```python
from build123d import *

# Parameters (mm, degrees)
BOSS_EXTRUDE1_DEPTH = 5.9944
SKETCH2_R           = 4.7244
CUT_EXTRUDE1_DEPTH  = 6.9944
SKETCH3_W           = 38.1
SKETCH3_H           = 1.5875
CUT_EXTRUDE2_DEPTH  = 6.9944


with BuildPart() as part:
    # Sketch1 → Boss-Extrude1 (new body)
    with BuildSketch(Plane.XY):
        Polygon((0, 0), (-38.1, 0), (-38.1, 6.35), (-44.0944, 6.35), (-44.0944, 19.05), (-38.1, 19.05), (-38.1, 31.75), (-44.0944, 31.75), (-44.0944, 44.45), (-38.1, 44.45), (-38.1, 50.8), (0, 50.8), (0, 44.45), (5.9944, 44.45), (5.9944, 31.75), (0, 31.75), (0, 19.05), (5.9944, 19.05), (5.9944, 6.35), (0, 6.35), align=None)
    extrude(amount=BOSS_EXTRUDE1_DEPTH)

    # Sketch2 → Cut-Extrude1 (cut, through all)
    with BuildSketch(Plane.XY.offset(5.9944)):
        with Locations((-19.05, 31.75)):
            Circle(SKETCH2_R)
    extrude(amount=-CUT_EXTRUDE1_DEPTH, mode=Mode.SUBTRACT)

    # Sketch3 → Cut-Extrude2 (cut, through all)
    with BuildSketch(Plane.XY.offset(5.9944)):
        with Locations((-19.05, 0.79375)):
            Rectangle(SKETCH3_W, SKETCH3_H)
        with Locations((-19.05, 50.00625)):
            Rectangle(SKETCH3_W, SKETCH3_H)
    extrude(amount=-CUT_EXTRUDE2_DEPTH, mode=Mode.SUBTRACT)


solid = part.part
```
Source: CAD feature listing. Evaluate the final solid. Frame: model axes, mm. A direction names the side the tool comes from. Round coordinates to 2 decimals unless told otherwise and drop trailing zeros. Write each loop counter-clockwise with the first axis right and the second up, starting at its lowest first coordinate (ties: lowest second). Pieces come first, ordered by that corner, then holes. Notation, with made-up numbers: M 62.25,78 L 91.25,78 A24 cw 91.25,100 Z; hole C 84,60 d4. An arc over 180 degrees is marked long. Answer as a JSON object with one key per item and string values. Group by question number.
(1) Section query B-B on x = -19.05. Output: boundary loops of the cut face in (y, z).
(2) Section query D-D on y = 5.5. Output: boundary loops of the cut face in (x, z).
(3) Reachability of faces 1 (the flat face through (-41, 31.75, 3)), 2 (the flat face through (-38.1, 47, 3)), 3 (the flat face through (3, 19.05, 3)) from +Z, -Z, +X, -X, +Y, -Y: full face, straight path, thin tool, end or side. Return the list, or none.
(4) Section query A-A on z = 1.8. Output: boundary loops of the cut face in (x, y), then the cut area to 3 significant figures.
(5) Section query C-C on y = 34. Output: boundary loops of the cut face in (x, z), then the cut area to 3 significant figures.
(6) First-contact query: pin 1 (3 mm diameter, centred on x = 3.5, z = 3.5, fed in from -Y); pin 2 (3 mm diameter, centred on x = -40.5, z = 3, fed in from +Y); pin 3 (15 mm diameter, centred on x = -19.05, y = 31.75, fed in from +Z); pin 4 (2.5 mm diameter, centred on y = 5, z = 4, fed in from +X). Flat tips, straight axial feed; report the tip coordinate or a pass-through.
(7) Mould query, pull axis Y, two halves, no side actions, for faces 4 (the flat face through (-41, 19.05, 3)), 5 (the flat face through (3, 31.75, 3)), 6 (the flat face through (3, 6.35, 3)), 7 (the flat face through (0, 4, 3)). Classes: +Y half, -Y half, draft (parallel to the pull), parting line (faces both ways), or undercut.
(8) Ray query, line 1 (Y direction, x = 3.5, z = 1.9); line 2 (Y direction, x = -19.05, z = 3.35); line 3 (X direction, y = 32, z = 5.45). Return the intervals inside material, ascending. Write a range as [from, to].
Computed values:
{
 "1": {"outline": "M 1.59,0 L 27.03,0 L 27.03,5.99 L 1.59,5.99 Z; M 36.47,0 L 49.21,0 L 49.21,5.99 L 36.47,5.99 Z"},
 "2": {"outline": "M -38.1,0 L 0,0 L 0,5.99 L -38.1,5.99 Z"},
 "3": {"face 1": "+Z, -Z, -X", "face 2": "+Z, -Z, -X, +Y", "face 3": "+Z, -Z, +X"},
 "4": {"outline": "M -44.09,6.35 L -38.1,6.35 L -38.1,1.59 L 0,1.59 L 0,6.35 L 5.99,6.35 L 5.99,19.05 L 0,19.05 L 0,31.75 L 5.99,31.75 L 5.99,44.45 L 0,44.45 L 0,49.21 L -38.1,49.21 L -38.1,44.45 L -44.09,44.45 L -44.09,31.75 L -38.1,31.75 L -38.1,19.05 L -44.09,19.05 Z; hole C -19.05,31.75 d9.45", "area": "2,050 mm^2"},
 "5": {"outline": "M -44.09,0 L -23.2,0 L -23.2,5.99 L -44.09,5.99 Z; M -14.9,0 L 5.99,0 L 5.99,5.99 L -14.9,5.99 Z", "area": "250 mm^2"},
 "6": {"pin 1": "y = 6.35", "pin 2": "y = 44.45", "pin 3": "z = 5.99", "pin 4": "x = 0"},
 "7": {"face 4": "undercut", "face 5": "undercut", "face 6": "-Y half", "face 7": "draft"},
 "8": {"line 1": "[6.35, 19.05], [31.75, 44.45]", "line 2": "[1.59, 27.03], [36.47, 49.21]", "line 3": "[-44.09, -23.77], [-14.33, 5.99]"}
}
